from build123d import *

# Parameters (mm, degrees)
F0_R     = 37
F0_R_2   = 3.25
F0_R_3   = 16
F1_DEPTH = 4
F2_SIZE  = 2.75
F3_SIZE  = 0.5


with BuildPart() as f1:
    # F0 (on Top) → F1 (new body)
    with BuildSketch(Plane.XY):
        Circle(F0_R)
        with Locations((0, -29)):
            Circle(F0_R_2, mode=Mode.SUBTRACT)
        with Locations((-29, 0)):
            Circle(F0_R_2, mode=Mode.SUBTRACT)
        Circle(F0_R_3, mode=Mode.SUBTRACT)
        with Locations((29, 0)):
            Circle(F0_R_2, mode=Mode.SUBTRACT)
        with Locations((0, 29)):
            Circle(F0_R_2, mode=Mode.SUBTRACT)
    extrude(amount=F1_DEPTH)

    # F2
    f2_edges = [f1.edges().sort_by_distance(p)[0] for p in [
        (-3.25, -29, 4),
        (-32.25, 0, 4),
        (-3.25, 29, 4),
        (25.75, 0, 4),
    ]]
    chamfer(f2_edges, length=F2_SIZE)

    # F3
    f3_edges = [f1.edges().sort_by_distance(p)[0] for p in [
        (16, 0, 2),
        (-16, 0, 0),
        (-16, 0, 4),
        (37, 0, 2),
        (-37, 0, 0),
        (-37, 0, 4),
        (-3.25, -29, 0),
        (-32.25, 0, 0),
        (25.75, 0, 0),
        (-3.25, 29, 0),
    ]]
    chamfer(f3_edges, length=F3_SIZE)


solid = f1.part
For this review, take the finished solid that the model builds, in its own axes (mm). Round coordinates to 2 decimals unless told otherwise and drop trailing zeros. One line per item, written item: value. Start each with the question number.
Item 1: For L1, parallel to Y at x = 0, z = 1; L2, parallel to Y at x = 0, z = 2.4; L3, parallel to X at y = -5.5, z = 2.1, list the stretches that pass through material, from the lowest coordinate up.
Item 2: Take a section at A-A (x = 0). State how many separate pieces and enclosed holes the cut face has, plus the area to 3 significant figures.
Item 3: Clearance check with flat-ended pins moving along their axes: pin 1 Ø1.5 at (y, z) = (23.5, 1) entering from +X; pin 2 Ø6 at (x, y) = (-29, 0) entering from +Z; pin 3 Ø1.5 at (x, z) = (-13, 0.5) entering from +Y; pin 4 Ø1.5 at (x, z) = (19.5, 1.5) entering from -Y. State where each tip first meets the part, or that it passes through.
Item 4: The part is to be moulded in two halves that separate along Y. For faces 1 (the flat face through (16, -8, 4)), 2 (the conical face through (32.26, 1.03, 1.42)), 3 (the cylindrical face through (-8.02, -36.12, 1.98)), say which applies: +Y half, -Y half, draft (parallel to the pull), parting line (faces both ways), or undercut.
Answer below:
1. L1: y = -37 to -32.25, -25.75 to -16, 16 to 25.75, 32.25 to 37
1. L2: y = -37 to -33.4, -24.6 to -16, 16 to 24.6, 33.4 to 37
1. L3: x = -36.59 to -15.02, 15.02 to 36.59
2. separate pieces: 4
2. enclosed holes: 0
2. area: 99.4 mm2
3. pin 1: stops at x = 29.18
3. pin 2: passes through
3. pin 3: stops at y = 34.91
3. pin 4: stops at y = -31.9
4. face 1: draft
4. face 2: undercut
4. face 3: parting line
